from build123d import *

# Parameters (mm, degrees)
SKETCH1_W            = 25
SKETCH1_H            = 34
BOSS_EXTRUDE2_DEPTH  = 4
SKETCH2_R            = 1.5
BOSS_EXTRUDE3_DEPTH  = 5
SKETCH3_R            = 1.5
BOSS_EXTRUDE4_DEPTH  = 2
SKETCH5_W            = 25
SKETCH5_H            = 4
BOSS_EXTRUDE5_DEPTH  = 55
SKETCH6_R            = 1.5
SKETCH6_W            = 25
SKETCH6_H            = 4
BOSS_EXTRUDE6_DEPTH  = 4
SKETCH7_W            = 4
SKETCH7_H            = 80
BOSS_EXTRUDE7_DEPTH  = 4
CUT_EXTRUDE2_DEPTH   = 5
SKETCH10_R           = 2
CUT_EXTRUDE3_DEPTH   = 1.5
SKETCH11_R           = 2
CUT_EXTRUDE4_DEPTH   = 1.5
SKETCH14_W           = 20
SKETCH14_H           = 18
BOSS_EXTRUDE8_DEPTH  = 4
SKETCH15_W           = 5
SKETCH15_H           = 18
BOSS_EXTRUDE9_DEPTH  = 29
SKETCH6_3_R          = 1.5
CUT_EXTRUDE5_DEPTH   = 35
FILLET2_R            = 2
SKETCH16_W           = 20
SKETCH16_H           = 18
BOSS_EXTRUDE10_DEPTH = 4
BOSS_EXTRUDE11_REACH = 35
SKETCH17_W           = 5
SKETCH17_H           = 18
FILLET3_R            = 2
SKETCH18_R           = 1.55
CUT_EXTRUDE6_DEPTH   = 5


with BuildPart() as part:
    # Sketch1 → Boss-Extrude2 (new body)
    with BuildSketch(Plane(origin=(0, 0, 0), x_dir=(1, 0, 0), z_dir=(0, 1, 0))):
        with Locations((12.5, -17)):
            Rectangle(SKETCH1_W, SKETCH1_H)
        with BuildLine():
            ThreePointArc((20.5, -15.95), (19.45, -17), (20.5, -18.05))
            ThreePointArc((20.5, -18.05), (21.55, -17), (20.5, -15.95))
        make_face(mode=Mode.SUBTRACT)
        with BuildLine():
            ThreePointArc((12.5, -26.05), (13.55, -25), (12.5, -23.95))
            ThreePointArc((12.5, -23.95), (11.45, -25), (12.5, -26.05))
        make_face(mode=Mode.SUBTRACT)
        with BuildLine():
            ThreePointArc((4.5, -15.95), (3.45, -17), (4.5, -18.05))
            ThreePointArc((4.5, -18.05), (5.55, -17), (4.5, -15.95))
        make_face(mode=Mode.SUBTRACT)
        with BuildLine():
            ThreePointArc((12.5, -7.95), (11.45, -9), (12.5, -10.05))
            ThreePointArc((12.5, -10.05), (13.55, -9), (12.5, -7.95))
        make_face(mode=Mode.SUBTRACT)
    extrude(amount=BOSS_EXTRUDE2_DEPTH)

    # Sketch2 → Boss-Extrude3 (add)
    with BuildSketch(Plane(origin=(0, 0, 0), x_dir=(-1, 0, 0), z_dir=(0, 0, -1))):
        Polygon((-25, 0), (0, 0), (4, 0), (4, 18), (-29, 18), (-29, 0), align=None)
        with Locations((-23.5, 13)):
            Circle(SKETCH2_R, mode=Mode.SUBTRACT)
        with Locations((-1.5, 13)):
            Circle(SKETCH2_R, mode=Mode.SUBTRACT)
    extrude(amount=-BOSS_EXTRUDE3_DEPTH)

    # Sketch3 → Boss-Extrude4 (add)
    with BuildSketch(Plane(origin=(0, 0, 0), x_dir=(-1, 0, 0), z_dir=(0, 0, -1))):
        with Locations((-1.5, 13)):
            Circle(SKETCH3_R)
        with Locations((-23.5, 13)):
            Circle(SKETCH3_R)
    extrude(amount=-BOSS_EXTRUDE4_DEPTH)

    # Sketch5 → Boss-Extrude5 (add)
    with BuildSketch(Plane.XY.offset(34)):
        with Locations((12.5, 2)):
            Rectangle(SKETCH5_W, SKETCH5_H)
    extrude(amount=BOSS_EXTRUDE5_DEPTH)

    # Sketch6 → Boss-Extrude6 (add)
    with BuildSketch(Plane.XY.offset(89)):
        Polygon((-4, 18), (29, 18), (29, 0), (25, 0), (25, 4), (0, 4), (0, 0), (-4, 0), align=None)
        with Locations((23.5, 13)):
            Circle(SKETCH6_R, mode=Mode.SUBTRACT)
        with Locations((1.5, 13)):
            Circle(SKETCH6_R, mode=Mode.SUBTRACT)
        with Locations((12.5, 2)):
            Rectangle(SKETCH6_W, SKETCH6_H)
    extrude(amount=-BOSS_EXTRUDE6_DEPTH)

    # Sketch7 → Boss-Extrude7 (add)
    with BuildSketch(Plane(origin=(0, 0, 0), x_dir=(-1, 0, 0), z_dir=(0, -1, 0))):
        with Locations((2, -45)):
            Rectangle(SKETCH7_W, SKETCH7_H)
        with Locations((-27, -45)):
            Rectangle(SKETCH7_W, SKETCH7_H)
    extrude(amount=-BOSS_EXTRUDE7_DEPTH)

    # Sketch9 → Cut-Extrude2 (cut, through all)
    with BuildSketch(Plane(origin=(0, 4, 0), x_dir=(1, 0, 0), z_dir=(0, 1, 0))):
        with BuildLine():
            ThreePointArc((1.95, -59), (3, -60.05), (4.05, -59))
            ThreePointArc((4.05, -59), (3, -57.95), (1.95, -59))
        make_face()
        with BuildLine():
            ThreePointArc((12.05, -59), (11, -57.95), (9.95, -59))
            ThreePointArc((9.95, -59), (11, -60.05), (12.05, -59))
        make_face()
        with BuildLine():
            ThreePointArc((12.05, -75), (11, -73.95), (9.95, -75))
            ThreePointArc((9.95, -75), (11, -76.05), (12.05, -75))
        make_face()
        with BuildLine():
            ThreePointArc((4.05, -75), (3, -73.95), (1.95, -75))
            ThreePointArc((1.95, -75), (3, -76.05), (4.05, -75))
        make_face()
    extrude(amount=-CUT_EXTRUDE2_DEPTH, mode=Mode.SUBTRACT)

    # Sketch10 → Cut-Extrude3 (cut)
    with BuildSketch(Plane(origin=(0, 4, 0), x_dir=(1, 0, 0), z_dir=(0, 1, 0))):
        with Locations((11, -75)):
            Circle(SKETCH10_R)
        with Locations((3, -75)):
            Circle(SKETCH10_R)
        with Locations((11, -59)):
            Circle(SKETCH10_R)
        with Locations((3, -59)):
            Circle(SKETCH10_R)
    extrude(amount=-CUT_EXTRUDE3_DEPTH, mode=Mode.SUBTRACT)

    # Sketch11 → Cut-Extrude4 (cut)
    with BuildSketch(Plane(origin=(0, 4, 0), x_dir=(1, 0, 0), z_dir=(0, 1, 0))):
        with Locations((4.5, -17)):
            Circle(SKETCH11_R)
        with Locations((12.5, -25)):
            Circle(SKETCH11_R)
        with Locations((20.5, -17)):
            Circle(SKETCH11_R)
        with Locations((12.5, -9)):
            Circle(SKETCH11_R)
    extrude(amount=-CUT_EXTRUDE4_DEPTH, mode=Mode.SUBTRACT)

    # Sketch14 → Boss-Extrude8 (add)
    with BuildSketch(Plane(origin=(29, 0, 0), x_dir=(0, 0, -1), z_dir=(1, 0, 0))):
        with Locations((-99, 9)):
            Rectangle(SKETCH14_W, SKETCH14_H)
        with BuildLine():
            Line((-102.666213823, 7.113305627), (-99.566213823, 7.113305627))
            ThreePointArc((-99.566213823, 7.113305627), (-98.016213823, 5.563305627), (-99.566213823, 4.013305627))
            Line((-99.566213823, 4.013305627), (-102.666213823, 4.013305627))
            ThreePointArc((-102.666213823, 4.013305627), (-104.216213823, 5.563305627), (-102.666213823, 7.113305627))
        make_face(mode=Mode.SUBTRACT)
    extrude(amount=-BOSS_EXTRUDE8_DEPTH)

    # Sketch15 → Boss-Extrude9 (add)
    with BuildSketch(Plane.ZY.offset(4)):
        with Locations((91.5, 9)):
            Rectangle(SKETCH15_W, SKETCH15_H)
    extrude(amount=-BOSS_EXTRUDE9_DEPTH)

    # Sketch6<3> → Cut-Extrude5 (cut)
    with BuildSketch(Plane.XY.offset(89)):
        with Locations((23.5, 13)):
            Circle(SKETCH6_3_R)
        with Locations((1.5, 13)):
            Circle(SKETCH6_3_R)
    extrude(amount=CUT_EXTRUDE5_DEPTH, mode=Mode.SUBTRACT)

    # Fillet2
    fillet2_edges = [part.edges().sort_by_distance(p)[0] for p in [
        (27, 18, 109),
        (27, 0, 109),
    ]]
    fillet(fillet2_edges, radius=FILLET2_R)

    # Sketch16 → Boss-Extrude10 (add)
    with BuildSketch(Plane(origin=(29, 0, 0), x_dir=(0, 0, -1), z_dir=(1, 0, 0))):
        with Locations((10, 9)):
            Rectangle(SKETCH16_W, SKETCH16_H)
    extrude(amount=-BOSS_EXTRUDE10_DEPTH)

    # Sketch17 → Boss-Extrude11 (add, up to next)
    with BuildSketch(Plane.ZY.offset(4), mode=Mode.PRIVATE) as boss_extrude11_sk1:
        with Locations((-2.5, 9)):
            Rectangle(SKETCH17_W, SKETCH17_H)
    boss_extrude11_tool1 = extrude(boss_extrude11_sk1.sketch, amount=-BOSS_EXTRUDE11_REACH, mode=Mode.PRIVATE) - part.part
    add(boss_extrude11_tool1.solids().sort_by_distance((-4, 9, -2.5))[0])

    # Fillet3
    fillet3_edges = [part.edges().sort_by_distance(p)[0] for p in [
        (27, 18, -20),
        (27, 0, -20),
    ]]
    fillet(fillet3_edges, radius=FILLET3_R)

    # Sketch18 → Cut-Extrude6 (cut, through all)
    with BuildSketch(Plane.ZY.offset(-25)):
        with Locations((-11.904808502, 5.295848229)):
            Circle(SKETCH18_R)
    extrude(amount=-CUT_EXTRUDE6_DEPTH, mode=Mode.SUBTRACT)


solid = part.part
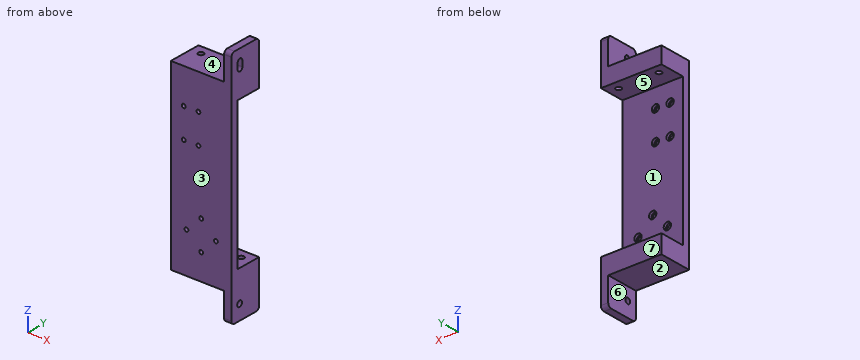
For this review, take the finished solid that the model builds, in its own axes (mm). Face numbers are marked on the shaded views. A direction names the side the tool comes from. Round coordinates to 2 decimals unless told otherwise and drop trailing zeros. Order: outer loops, then holes, each group sorted by start corner. A loop starts at its lowest first (then second) coordinate and runs counter-clockwise, first axis right, second up. Notation, with made-up numbers: (22.5, -1) -> (77.5, -1) arc R18 ccw to (77.5, 16) -> close; hole circle Ø8 at (13.5, 33.5). An arc over 180 degrees is marked (long way). Put each result on its own line as item: value.
Q1. Add section A-A on z = 90.5. Write out the cut boundary in (x, y), plus the area to 3 significant figures.
Check result:
outline: (-4, 0) -> (29, 0) -> (29, 18) -> (-4, 18) -> close; hole circle Ø3 at (1.5, 13); hole circle Ø3 at (23.5, 13)
area: 580 mm2
Q2. Insertion check: pin 1 Ø4 at (x, y) = (18, 15.5) entering from -Z; pin 2 Ø6 at (x, y) = (13.5, 10) entering from +Z; pin 3 Ø4.5 at (y, z) = (10.5, 104.5) entering from -X. Each pin has a flat end and moves straight along its axis. Give the tip position at first contact, or say it passes through.
Check result:
pin 1: z = -5
pin 2: z = 94
pin 3: x = 25
Q3. Mouldability with a two-part tool opening along Z and no side actions: class the marked faces 1, 2 and 3 as pulls with the +Z half, pulls with the -Z half, needs draft (parallel to the pull), parting line crosses it, or undercut.
Check result:
face 1: undercut
face 2: pulls with the -Z half
face 3: needs draft
Q4. Add section B-B on z = 30. Write out the cut boundary in (x, y), plus the area to 3 significant figures.
Check result:
outline: (-4, 0) -> (29, 0) -> (29, 4) -> (-4, 4) -> close
area: 132 mm2
Q5. Machinability: for the marked faces 4, 5, 6 and 7, which of the approach directions +Z, -Z, +X, -X, +Y, -Y give a long, thin tool a straight path to every point of the face, cutting with its end or side? Answer none if there is none.
Check result:
face 4: +Z, -X, +Y, -Y
face 5: +X, -X, +Y
face 6: -Z, -X, +Y, -Y
face 7: +Z, -Z, +X, -X, +Y
Q6. For probe 1 along X at (y, z) = (2.95, 59); probe 2 along X at (y, z) = (0.8, 25); probe 3 along Z at (x, y) = (11, 7), list the stretches that pass through material, from the lowest coordinate up. Write a range as [from, to].
Check result:
probe 1: [-4, 1], [5, 9], [13, 29]
probe 2: [-4, 11.45], [13.55, 29]
probe 3: [-5, 5], [85, 94]
